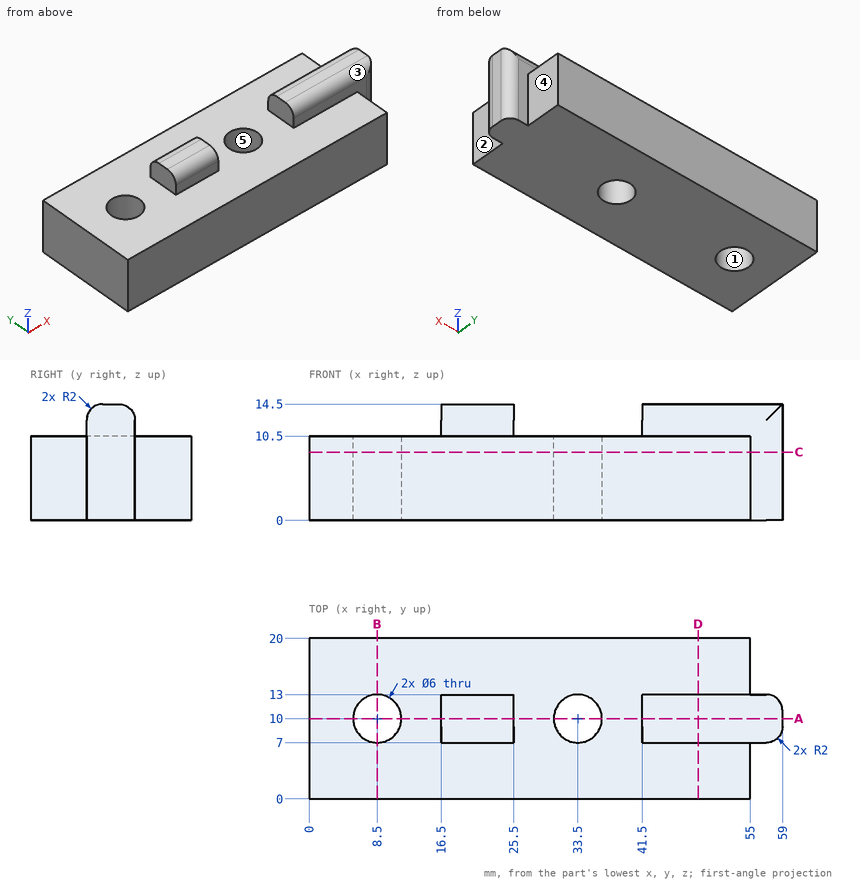
Study the drawing (mm; zero at the part's minimum x, y, z) and answer. A direction names the side the tool comes from. Coordinates: 2 decimals unless noted, no trailing zeros. Write each loop counter-clockwise with the first axis right and the second up, starting at its lowest first coordinate (ties: lowest second). Pieces come first, ordered by that corner, then holes. Notation, with made-up numbers: (29, -21.5) - (82, -21.5) arc R25 ccw to (82, 0.5) - close; hole circle Ø9 at (-10, 88.25). An arc over 180 degrees is marked (long way). One line per item, written item: value.
1) Find section C-C (z = 8.5). Give the vertices of the cut face in (x, y).
Geometry check:
outline: (0, 0) - (55, 0) - (55, 7) - (57, 7) arc R2 ccw to (59, 9) - (59, 11) arc R2 ccw to (57, 13) - (55, 13) - (55, 20) - (0, 20) - close; hole circle Ø6 at (8.5, 10); hole circle Ø6 at (33.5, 10)
2) Find section B-B (x = 8.5). Give the vertices of the cut face in (y, z), and give its area (3 significant figures).
Geometry check:
outline: (0, 0) - (7, 0) - (7, 10.5) - (0, 10.5) - close; (13, 0) - (20, 0) - (20, 10.5) - (13, 10.5) - close
area: 147 mm2
3) Each of these flat-tipped pins is pushed along its axis until it touches: pin 1 Ø7.5 at (y, z) = (15, 7.5) entering from +X; pin 2 Ø6 at (x, y) = (49.5, 15) entering from +Z; pin 3 Ø1.6 at (x, z) = (22.5, 12) entering from +Y. Where does it stop, or does it pass through?
Geometry check:
pin 1: stops at x = 58.98
pin 2: stops at z = 14.23
pin 3: stops at y = 13
4) Find section D-D (x = 48.5). Give the vertices of the cut face in (y, z), and give its area (3 significant figures).
Geometry check:
outline: (0, 0) - (20, 0) - (20, 10.5) - (13, 10.5) - (13, 12.5) arc R2 ccw to (11, 14.5) - (9, 14.5) arc R2 ccw to (7, 12.5) - (7, 10.5) - (0, 10.5) - close
area: 232 mm2
5) Consider line 1 along Y through (x, z) = (8.5, 3); line 2 along X through (y, z) = (9.75, 12.25); line 3 along X through (y, z) = (14.25, 9.25). Determine where each line is inside the solid, lowest interval first. Write a range as from..to.
Geometry check:
line 1: y = 0..7, 13..20
line 2: x = 16.5..25.5, 41.5..59
line 3: x = 0..55
6) A tool of negligible diameter and unlimited length cuts with its end or side. For the marked faces 1 and 2, from which of +Z, -Z, +X, -X, +Y, -Y can it reach the whole face along a straight path? Write none if from no direction.
Geometry check:
face 1: +Z, -Z
face 2: +Z, -Z, +X, -Y
7) For a pull along X with two mould halves and no side action, classify the marked faces 3, 4 and 5 as pulls with the +X half, pulls with the -X half, needs draft (parallel to the pull), parting line crosses it, or undercut.
Geometry check:
face 3: needs draft
face 4: pulls with the +X half
face 5: undercut
8) Find section A-A (y = 10). Give the vertices of the cut face in (x, z), and give its area (4 significant figures).
Geometry check:
outline: (0, 0) - (5.5, 0) - (5.5, 10.5) - (0, 10.5) - close; (11.5, 0) - (30.5, 0) - (30.5, 10.5) - (25.5, 10.5) - (25.5, 14.5) - (16.5, 14.5) - (16.5, 10.5) - (11.5, 10.5) - close; (36.5, 0) - (59, 0) - (59, 14.5) - (41.5, 14.5) - (41.5, 10.5) - (36.5, 10.5) - close
area: 599.5 mm2
